Could you check a few things on this model? Use its own coordinates, in mm. Face numbers are marked on the shaded views. A direction names the side the tool comes from. Coordinates: 2 decimals unless noted, no trailing zeros. Loops run counter-clockwise (first coordinate to the right, second up) from the corner with the lowest first, then second, coordinate; pieces in that order, holes last.
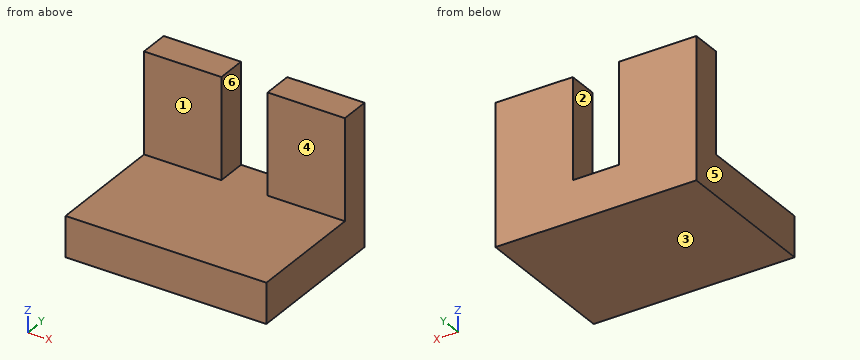
Autodesk Inventor part; units mm, degrees
ref_plane "YZ Plane" through (0, 0, 0) normal (1, 0, 0) x (0, 1, 0)
ref_plane "XZ Plane" through (0, 0, 0) normal (0, 1, 0) x (-1, 0, 0)
ref_plane "XY Plane" through (0, 0, 0) normal (0, 0, 1) x (1, 0, 0)
sketch "Sketch1" plane through (0, 0, 0) normal (0, 0, 1) x (1, 0, 0)
  line L0 (0, 0) -> (25.4, 0)
  line L1 (25.4, 0) -> (25.4, -19.05)
  line L2 (25.4, -19.05) -> (0, -19.05)
  line L3 (0, -19.05) -> (0, 0)
  dimension "d0" = 25.4
  dimension "d1" = 19.05
extrude "Extrusion1" add sketch "Sketch1" along normal blind 5.08
sketch "Sketch2" plane through (0, 0, 5.08) normal (0, 0, 1) x (1, 0, 0)
  line L0 (25.4, 0) -> (0, 0)
  line L1 (0, 0) -> (9.779, 0)
  line L2 (9.779, 0) -> (9.779, -3.81)
  line L3 (9.779, -3.81) -> (0, -3.81)
  line L4 (0, -3.81) -> (0, 0)
  line L5 (25.4, 0) -> (15.621, 0)
  line L6 (15.621, 0) -> (15.621, -3.81)
  line L7 (15.621, -3.81) -> (25.4, -3.81)
  line L8 (25.4, -3.81) -> (25.4, 0)
  dimension "d4" = 9.779
  dimension "d5" = 3.81
  dimension "d6" = 9.779
extrude "Extrusion2" add sketch "Sketch2" along normal blind 12.7
(1) We'd pull the mould along X, two halves only. Please class the marked faces 4, 5 and 6: +X half, -X half, draft (parallel to the pull), parting line (faces both ways), or undercut.
Answers:
face 4: draft
face 5: -X half
face 6: undercut
(2) Which directions (+Z, -Z, +X, -X, +Y, -Y) give clear straight access to the entire face, cutting with the end or side of a thin tool? Please do the marked faces 1, 2 and 3.
Answers:
face 1: +Z, +X, -X, -Y
face 2: +Z, +Y, -Y
face 3: -Z, +X, -X, +Y, -Y
(3) Imagine slicing it at A-A, the plane z = 10.5. Write out the boundary of the cut face in (x, y).
Answers:
outline: (0, -3.81) - (9.78, -3.81) - (9.78, 0) - (0, 0) - close; (15.62, -3.81) - (25.4, -3.81) - (25.4, 0) - (15.62, 0) - close
(4) For pin 1 (6 mm diameter, centred on x = 15, z = 11.5, fed in from -Y); pin 2 (8 mm diameter, centred on x = 14, y = -14, fed in from +Z), each with a flat end and sliding along its axis, tell me the tip position at first contact or that it passes through.
Answers:
pin 1: stops at y = -3.81
pin 2: stops at z = 5.08
(5) I need wall thicknesses on probe 1 along X at (y, z) = (-3.25, 10.75); probe 2 along Z at (x, y) = (17.75, -16.25); probe 3 along Y at (x, z) = (1.75, 17). Which ranges of each line are inside material? Lowest first, please.
Answers:
probe 1: x = 0 to 9.78, 15.62 to 25.4
probe 2: z = 0 to 5.08
probe 3: y = -3.81 to 0
(6) Imagine slicing it at C-C, the plane x = 5.25. Write out the boundary of the cut face in (y, z), and give its area (3 significant figures).
Answers:
outline: (-19.05, 0) - (0, 0) - (0, 17.78) - (-3.81, 17.78) - (-3.81, 5.08) - (-19.05, 5.08) - close
area: 145 mm2
(7) Imagine slicing it at B-B, the plane y = -1.5. Write out the boundary of the cut face in (x, z).
Answers:
outline: (0, 0) - (25.4, 0) - (25.4, 17.78) - (15.62, 17.78) - (15.62, 5.08) - (9.78, 5.08) - (9.78, 17.78) - (0, 17.78) - close
(8) Imagine slicing it at D-D, the plane y = -7. Write out the boundary of the cut face in (x, z), and give its area (3 significant figures).
Answers:
outline: (0, 0) - (25.4, 0) - (25.4, 5.08) - (0, 5.08) - close
area: 129 mm2
